Build history of the part. All positions in model axes, mm. Give positions to 0.01 mm unless a question says otherwise; leave off trailing zeros. Write each loop counter-clockwise with the first axis right and the second up, starting at its lowest first coordinate (ties: lowest second). Pieces come first, ordered by that corner, then holes. Notation, with made-up numbers: (79, -35.5) -> (129, -35.5) arc R13 cw to (129, -29.5) -> close; hole circle Ø7 at (48.5, 28). An arc over 180 degrees is marked (long way). Put each result on its own line as item: value.
from build123d import *

# Parameters (mm, degrees)
F1_DEPTH = 26


with BuildPart() as f1:
    # F0 (on Front) → F1 (new body)
    with BuildSketch(Plane.XZ):
        with BuildLine():
            Line((-500, 181.940629), (-500, -181.940629))
            ThreePointArc((-500, -181.940629), (-487.887011, -214.568446), (-457.417023, -231.387447))
            Line((-457.417023, -231.387447), (-89.004272, -286.649359))
            ThreePointArc((-89.004272, -286.649359), (0, -293.287548), (89.004272, -286.649359))
            Line((89.004272, -286.649359), (457.417023, -231.387447))
            ThreePointArc((457.417023, -231.387447), (487.887011, -214.568446), (500, -181.940629))
            Line((500, -181.940629), (500, 181.940629))
            ThreePointArc((500, 181.940629), (487.887011, 214.568446), (457.417023, 231.387447))
            Line((457.417023, 231.387447), (89.004272, 286.649359))
            ThreePointArc((89.004272, 286.649359), (0, 293.287548), (-89.004272, 286.649359))
            Line((-89.004272, 286.649359), (-457.417023, 231.387447))
            ThreePointArc((-457.417023, 231.387447), (-487.887011, 214.568446), (-500, 181.940629))
        make_face()
        Polygon((-246.29619, 123.066799), (0, 14.747886), (246.29619, 123.066799), (257.16581, 98.351391), (33.53383, 0), (257.16581, -98.351391), (246.29619, -123.066799), (0, -14.747886), (-246.29619, -123.066799), (-257.16581, -98.351391), (-33.53383, 0), (-257.16581, 98.351391), align=None, mode=Mode.SUBTRACT)
    extrude(amount=F1_DEPTH)


solid = f1.part
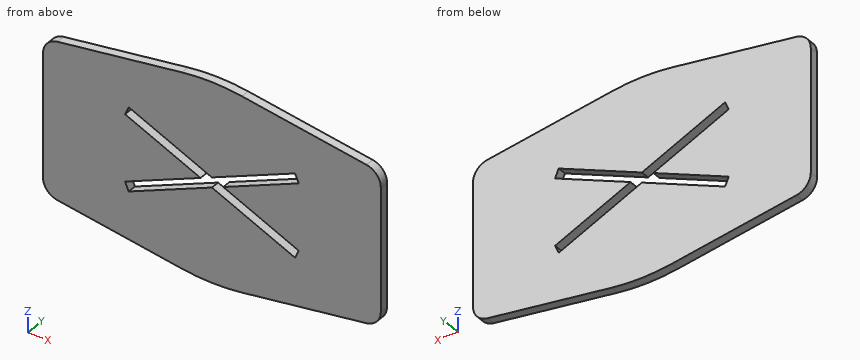
1) Slice it at A-A (y = -8.25). Write the cut outline in (x, z).
Filled sheet:
outline: (-500, -181.94) arc R50 ccw to (-457.42, -231.39) -> (-89, -286.65) arc R600 ccw to (89, -286.65) -> (457.42, -231.39) arc R50 ccw to (500, -181.94) -> (500, 181.94) arc R50 ccw to (457.42, 231.39) -> (89, 286.65) arc R600 ccw to (-89, 286.65) -> (-457.42, 231.39) arc R50 ccw to (-500, 181.94) -> close; hole (-257.17, -98.35) -> (-246.3, -123.07) -> (0, -14.75) -> (246.3, -123.07) -> (257.17, -98.35) -> (33.53, 0) -> (257.17, 98.35) -> (246.3, 123.07) -> (0, 14.75) -> (-246.3, 123.07) -> (-257.17, 98.35) -> (-33.53, 0) -> close
2) Slice it at C-C (x = -160). Write the cut outline in (y, z).
Filled sheet:
outline: (-26, -276) -> (0, -276) -> (0, -85.11) -> (-26, -85.11) -> close; (-26, -55.62) -> (0, -55.62) -> (0, 55.62) -> (-26, 55.62) -> close; (-26, 85.11) -> (0, 85.11) -> (0, 276) -> (-26, 276) -> close
3) Slice it at B-B (x = 14.5). Write the cut outline in (y, z).
Filled sheet:
outline: (-26, -293.11) -> (0, -293.11) -> (0, -21.12) -> (-26, -21.12) -> close; (-26, 21.12) -> (0, 21.12) -> (0, 293.11) -> (-26, 293.11) -> close
4) Pin check, flat tips, straight feed: pin 1 (1.5 mm diameter, centred on x = -393.5, z = 72, fed in from +Y); pin 2 (8 mm diameter, centred on x = -77, y = -18, fed in from +Z); pin 3 (10 mm diameter, centred on x = 224.5, y = -9, fed in from +Z) (3 decimals); pin 4 (4 mm diameter, centred on x = 148, y = -16.5, fed in from +Z). Stop position of each tip, or through.
Filled sheet:
pin 1: y = 0
pin 2: z = 288.83
pin 3: z = 267.075
pin 4: z = 278.1
5) Slice it at D-D (z = 26.5). Write the cut outline in (x, y), plus the area to 3 significant figures.
Filled sheet:
outline: (-500, -26) -> (-93.79, -26) -> (-93.79, 0) -> (-500, 0) -> close; (-26.72, -26) -> (26.72, -26) -> (26.72, 0) -> (-26.72, 0) -> close; (93.79, -26) -> (500, -26) -> (500, 0) -> (93.79, 0) -> close
area: 22,500 mm2
6) Wall check: L1, parallel to Z at x = 225.5, y = -15.5 (3 decimals); L2, parallel to X at y = -22, z = 100; L3, parallel to Z at x = 221, y = -19.25. Give the ranges that are in metal, low to high.
Filled sheet:
L1: -266.175 to -113.921, -84.425 to 84.425, 113.921 to 266.175
L2: -500 to -256.44, -193.85 to 193.85, 256.44 to 500
L3: -266.85 to -111.94, -82.45 to 82.45, 111.94 to 266.85
